Read the model definition and answer for the solid it produces. Units are mm, in the model's axes. Round coordinates to 2 decimals unless told otherwise and drop trailing zeros. Write each loop counter-clockwise with the first axis right and the second up, starting at its lowest first coordinate (ties: lowest second). Pieces come first, ordered by that corner, then holes.
from build123d import *

# Parameters (mm, degrees)
BOSS_EXTRUDE1_DEPTH = 6.35
BOSS_EXTRUDE2_DEPTH = 6.35


with BuildPart() as part:
    # Sketch1 → Boss-Extrude1 (new body)
    with BuildSketch(Plane(origin=(0, 0, 0), x_dir=(0, 0, -1), z_dir=(1, 0, 0))):
        with BuildLine():
            Line((-106.172, 0), (-62.992, 43.18))
            Line((-62.992, 43.18), (0, 43.18))
            Line((0, 43.18), (0, 40.64))
            ThreePointArc((0, 40.64), (-6.479930943, 21.59), (0, 2.54))
            Line((0, 2.54), (0, 0))
            Line((0, 0), (-106.172, 0))
        make_face()
    extrude(amount=BOSS_EXTRUDE1_DEPTH)

    # Sketch2 → Boss-Extrude2 (add)
    with BuildSketch(Plane(origin=(6.35, 0, 0), x_dir=(0, 0, -1), z_dir=(1, 0, 0))):
        Polygon((-68.072, 0), (-169.672, 0), (-144.272, 10.16), (-68.072, 15.24), align=None)
    extrude(amount=-BOSS_EXTRUDE2_DEPTH)


solid = part.part
Q1. Section A-A (x = 4) is taken. Determine the outline of the cut face in (y, z).
Verdict:
outline: (0, 0) - (2.54, 0) arc R31.24 cw to (40.64, 0) - (43.18, 0) - (43.18, 62.99) - (13.61, 92.56) - (10.16, 144.27) - (0, 169.67) - close
Q2. Straight lines are drawn through the part: probe 1 along Z at (x, y) = (3.25, 36.5); probe 2 along Z at (x, y) = (5.25, 32.5); probe 3 along Y at (x, z) = (1.25, 105). For each, find the intervals that lie inside material, in ascending order.
Verdict:
probe 1: z = 2.69 to 69.67
probe 2: z = 4.51 to 73.67
probe 3: y = 0 to 12.78
Q3. Section B-B (z = 112.5) is taken. Determine the outline of the cut face in (x, y), then the cut area to 3 significant figures.
Verdict:
outline: (0, 0) - (6.35, 0) - (6.35, 12.28) - (0, 12.28) - close
area: 78.0 mm2
Q4. Section C-C (y = 31.5) is taken. Determine the outline of the cut face in (x, z).
Verdict:
outline: (0, 4.87) - (6.35, 4.87) - (6.35, 74.67) - (0, 74.67) - close
Q5. Determine the mould class of faces 1 (the flat face through (3, 43.18, 32)), 2 (the cylindrical face through (3.13, 21.88, 6.48)), 3 (the flat face through (3, 0, 84)) for opening direction Y: pulls with the +Y half, pulls with the -Y half, needs draft (parallel to the pull), parting line crosses it, or undercut.
Verdict:
face 1: pulls with the +Y half
face 2: undercut
face 3: pulls with the -Y half
